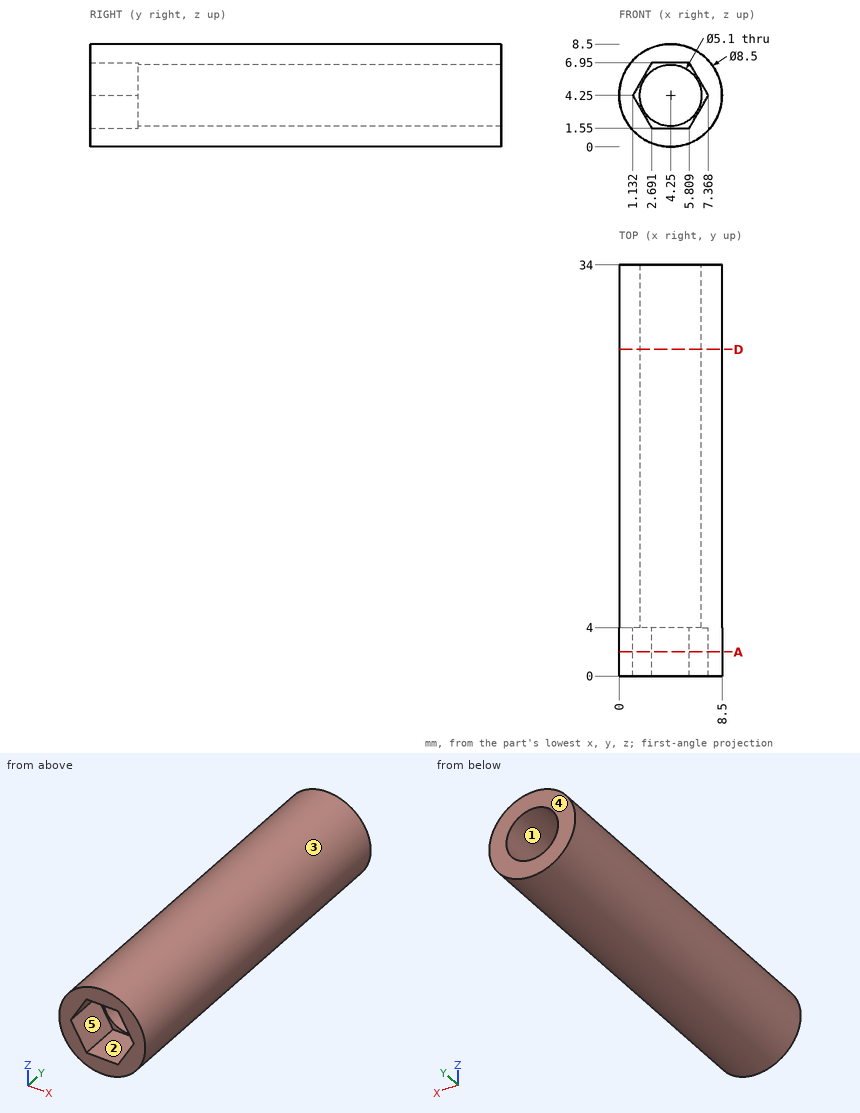
Verification items for this drawing (mm, ordinates from the low corner). A direction names the side the tool comes from. Coordinates: 2 decimals unless noted, no trailing zeros. Write each loop counter-clockwise with the first axis right and the second up, starting at its lowest first coordinate (ties: lowest second). Pieces come first, ordered by that corner, then holes. Notation, with made-up numbers: M 3,73 L 25,73 A20 cw 25,112 Z; hole C 77.5,33.25 d6. An arc over 180 degrees is marked long. Answer as a JSON object with one key per item and string values. Group by question number.
(1) Material ranges on line 1 (Z direction, x = 4.25, y = 21.75); line 2 (Z direction, x = 5.5, y = 19.5), recorded low to high.
(2) Tool access check on the marked faces 1 and 2. Record the directions out of +Z, -Z, +X, -X, +Y, -Y that give a thin tool (end or side, any length) a straight path to the whole face; none if there is none.
(3) Release check for a two-part mould opening along Z. For the marked faces 3, 4 and 5 record: +Z half, -Z half, draft (parallel to the pull), parting line (faces both ways), or undercut.
(4) Gauge pin test, flat ends, axial feed: pin 1 (1 mm diameter, centred on x = 3, y = 17, fed in from +Z); pin 2 (1 mm diameter, centred on y = 24, z = 1.5, fed in from +X) (1 decimal); pin 3 (0.9 mm diameter, centred on x = 5, y = 2.5, fed in from -Z). Record the tip position at first contact, or that the pin passes through.
(5) Cross-section at D-D, the plane y = 27. Record the cut outline in (x, z), and give its area (3 significant figures).
(6) Cross-section at A-A, the plane y = 2. Record the cut outline in (x, z), and give its area (3 significant figures).
Reply:
{
 "1": {"line 1": "0 to 1.7, 6.8 to 8.5", "line 2": "0.19 to 2.03, 6.47 to 8.31"},
 "2": {"face 1": "+Y, -Y", "face 2": "-Y"},
 "3": {"face 3": "parting line", "face 4": "draft", "face 5": "undercut"},
 "4": {"pin 1": "z = 8.43", "pin 2": "x = 7.9", "pin 3": "z = 0.01"},
 "5": {"outline": "C 4.25,4.25 d8.5; hole C 4.25,4.25 d5.1", "area": "36.3 mm²"},
 "6": {"outline": "C 4.25,4.25 d8.5; hole M 1.13,4.25 L 2.69,1.55 L 5.81,1.55 L 7.37,4.25 L 5.81,6.95 L 2.69,6.95 Z", "area": "31.5 mm²"}
}
